Geometry check sheet. Reference: the model listing, model coordinates, mm. Face numbers are marked on the shaded views. A direction names the side the tool comes from. Round coordinates to 2 decimals unless told otherwise and drop trailing zeros. Order: outer loops, then holes, each group sorted by start corner. A loop starts at its lowest first (then second) coordinate and runs counter-clockwise, first axis right, second up. Notation, with made-up numbers: (-36.75, -17.5) -> (10.25, -17.5) arc R28 ccw to (10.25, 21.5) -> close; hole circle Ø6 at (59.5, 56.25). An arc over 180 degrees is marked (long way). Use a Markdown table: item, result. Add a question column.
Item 1: Mould release check, pull along X, two halves, no side actions. Record for the marked faces 4, 5 and 6: pulls with the +X half, pulls with the -X half, needs draft (parallel to the pull), parting line crosses it, or undercut.
Item 2: Sectioned sample at C-C, the plane y = 66.5. Record the cut outline in (x, z), and give its area (3 significant figures).
Item 3: Sectioned sample at A-A, the plane z = 39. Record the cut outline in (x, y), and give its area (3 significant figures).
Item 4: Sectioned sample at D-D, the plane y = 80. Record the cut outline in (x, z).
Item 5: Sectioned sample at B-B, the plane x = 66.5. Record the cut outline in (y, z).
Item 6: Gauge pin test, flat ends, axial feed: pin 1 Ø7.5 at (x, z) = (83.5, 43.5) entering from +Y; pin 2 Ø20.5 at (y, z) = (89, 41.5) entering from +X; pin 3 Ø2 at (x, y) = (123, 21.5) entering from +Z. Record the tip position at first contact, or that the pin passes through.
Item 7: Set-up check for the marked faces 1, 2 and 3: record each of +Z, -Z, +X, -X, +Y, -Y from which the full face is reachable in a straight line by a thin tool's end or side.
Item 8: Material ranges on probe 1 along Z at (x, y) = (104.5, 81); probe 2 along Y at (x, z) = (44, 31), recorded low to high. Write a range as [from, to].
from build123d import *

# Parameters (mm, degrees)
F1_DEPTH = 101.6
F3_DEPTH = 25.4
F5_DEPTH = 25.4


with BuildPart() as f1:
    # F0 (on Front) → F1 (new body)
    with BuildSketch(Plane.XZ):
        Polygon((0, 50.8), (0, 0), (152.4, 0), (152.4, 25.4), (25.4, 25.4), (25.4, 50.8), align=None)
        Polygon((152.4, 25.4), (25.4, 50.8), (25.4, 25.4), align=None)
    extrude(amount=-F1_DEPTH)

    # F2 (on face) → F3 (cut)
    with BuildSketch(Plane.XZ):
        Polygon((152.4, 25.4), (25.4, 50.8), (25.4, 25.4), align=None)
    extrude(amount=-F3_DEPTH, mode=Mode.SUBTRACT)

    # F4 (on face) → F5 (cut)
    with BuildSketch(Plane(origin=(0, 101.6, 0), x_dir=(-1, 0, 0), z_dir=(0, 1, 0))):
        Polygon((-25.4, 25.4), (-25.4, 50.8), (-152.4, 25.4), align=None)
    extrude(amount=-F5_DEPTH, mode=Mode.SUBTRACT)


solid = f1.part
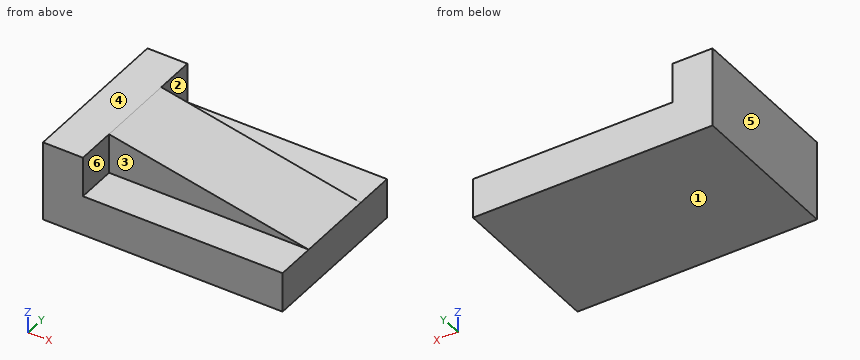
Found:
| question | item | result |
|---|---|---|
| 1 | face 4 | needs draft |
| 1 | face 5 | pulls with the -X half |
| 1 | face 6 | pulls with the +X half |
| 2 | outline | (0, 0) -> (152.4, 0) -> (152.4, 25.4) -> (25.4, 50.8) -> (0, 50.8) -> close |
| 2 | area | 6,130 mm2 |
| 3 | outline | (0, 0) -> (25.4, 0) -> (25.4, 25.4) -> (84.4, 25.4) -> (84.4, 76.2) -> (25.4, 76.2) -> (25.4, 101.6) -> (0, 101.6) -> close |
| 3 | area | 5,580 mm2 |
| 4 | outline | (0, 0) -> (152.4, 0) -> (152.4, 25.4) -> (25.4, 25.4) -> (25.4, 50.8) -> (0, 50.8) -> close |
| 5 | outline | (0, 0) -> (101.6, 0) -> (101.6, 25.4) -> (76.2, 25.4) -> (76.2, 42.58) -> (25.4, 42.58) -> (25.4, 25.4) -> (0, 25.4) -> close |
| 6 | pin 1 | passes through |
| 6 | pin 2 | stops at x = 25.4 |
| 6 | pin 3 | stops at z = 25.4 |
| 7 | face 1 | -Z, +X, -X, +Y, -Y |
| 7 | face 2 | +Z, +X, +Y |
| 7 | face 3 | +Z, +X, -Y |
| 8 | probe 1 | z = [0, 25.4] |
| 8 | probe 2 | y = [25.4, 76.2] |
